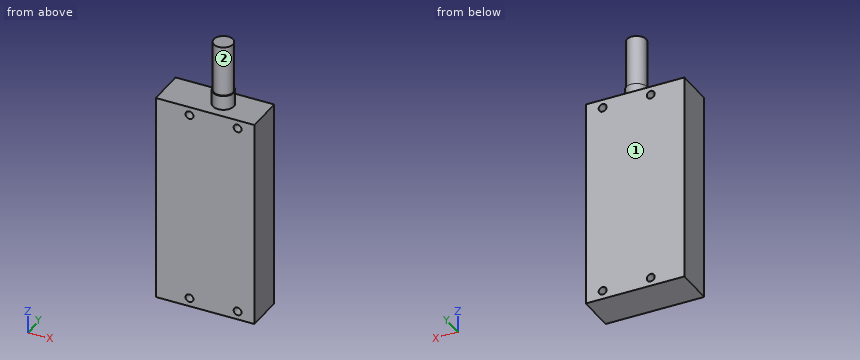
```python
from build123d import *

# Parameters (mm, degrees)
F0_W     = 41
F0_H     = 87
F1_DEPTH = 16
F3_D     = 3.3
F3_DEPTH = 27.7
F3_TIP   = 0.9914200214
F4_R     = 4.375
F5_DEPTH = 6
F6_R     = 4
F7_DEPTH = 21


with BuildPart() as f1:
    # F0 (on Front) → F1 (new body)
    with BuildSketch(Plane.XZ):
        with Locations((20.5, 43.5)):
            Rectangle(F0_W, F0_H)
    extrude(amount=F1_DEPTH)

    # F3
    with Locations(Plane.XZ.offset(16)):
        with Locations((14, 83.5), (34, 83.5), (14, 3.5), (34, 3.5)):
            Hole(F3_D / 2, depth=F3_DEPTH)
            with Locations((0, 0, -(F3_DEPTH + F3_TIP / 2))):  # 118° drill point
                Cone(0, F3_D / 2, F3_TIP, mode=Mode.SUBTRACT)

    # F4 (on face) → F5 (join)
    with BuildSketch(Plane.XY.offset(87)):
        with Locations((24, -8)):
            Circle(F4_R)
    extrude(amount=F5_DEPTH)

    # F6 (on face) → F7 (join)
    with BuildSketch(Plane.XY.offset(93)):
        with Locations((24, -8)):
            Circle(F6_R)
    extrude(amount=F7_DEPTH)


solid = f1.part
```
CAD build for the part. Positions are in the model's coordinates, mm. Face numbers are marked on the shaded views. A direction names the side the tool comes from. Give positions to 0.01 mm unless a question says otherwise; leave off trailing zeros. Write each loop counter-clockwise with the first axis right and the second up, starting at its lowest first coordinate (ties: lowest second). Pieces come first, ordered by that corner, then holes. Notation, with made-up numbers: M 87,11 L 124,11 A24 cw 124,29 Z; hole C -10.75,6.25 d5. An arc over 180 degrees is marked long. Return JSON: item names as keys, results as strings. Group by question number.
(1) Band-saw the part on B-B (z = 3.5). Give the cut face in (x, y), and give its area (3 significant figures).
(2) Drill centre lines: L1, parallel to Z at x = 14, y = -9.25; L2, parallel to X at y = -8.5, z = 83.5; L3, parallel to Z at x = 15, y = -3. Where is each one in solid material? Low to high. Write a range as [from, to].
(3) Flat gauge pins, fed straight in: pin 1 Ø1 at (y, z) = (-10.5, 88.5) entering from +X; pin 2 Ø1 at (x, y) = (12.5, -4) entering from +Z. Where does each tip first touch, or does it go through?
(4) Band-saw the part on C-C (y = -8). Give the cut face in (x, z) (3 decimals).
(5) 3-axis set-ups, long thin cutter, end or side, ignore diameter. For the marked faces 1 and 2: which of +Z, -Z, +X, -X, +Y, -Y reach the whole face in a straight line?
(6) Band-saw the part on D-D (x = 24). Give the cut face in (y, z) (3 decimals).
(7) Band-saw the part on A-A (x = 14). Give the cut face in (y, z), and give its area (3 significant figures).
Entries:
{
 "1": {"outline": "M 0,-16 L 12.35,-16 L 12.35,0 L 0,0 Z; M 15.65,-16 L 32.35,-16 L 32.35,0 L 15.65,0 Z; M 35.65,-16 L 41,-16 L 41,0 L 35.65,0 Z", "area": "550 mm^2"},
 "2": {"L1": "z = [0, 1.85], [5.15, 81.85], [85.15, 87]", "L2": "x = [0, 12.35], [15.65, 32.35], [35.65, 41]", "L3": "z = [0, 2.19], [4.81, 82.19], [84.81, 87]"},
 "3": {"pin 1": "stops at x = 27.89", "pin 2": "stops at z = 87"},
 "4": {"outline": "M 0,0 L 41,0 L 41,87 L 28.375,87 L 28.375,93 L 28,93 L 28,114 L 20,114 L 20,93 L 19.625,93 L 19.625,87 L 0,87 Z; hole C 14,3.5 d3.3; hole C 14,83.5 d3.3; hole C 34,3.5 d3.3; hole C 34,83.5 d3.3"},
 "5": {"face 1": "+Z, -Z, +X, -X, +Y", "face 2": "+Z"},
 "6": {"outline": "M -16,0 L 0,0 L 0,87 L -3.625,87 L -3.625,93 L -4,93 L -4,114 L -12,114 L -12,93 L -12.375,93 L -12.375,87 L -16,87 Z"},
 "7": {"outline": "M -16,0 L 0,0 L 0,1.85 L -16,1.85 Z; M -16,5.15 L 0,5.15 L 0,81.85 L -16,81.85 Z; M -16,85.15 L 0,85.15 L 0,87 L -16,87 Z", "area": "1,290 mm^2"}
}
